Source: CAD feature listing. Evaluate the final solid. Frame: model axes, mm. Face numbers are marked on the shaded views. A direction names the side the tool comes from. Coordinates: 2 decimals unless noted, no trailing zeros. Order: outer loops, then holes, each group sorted by start corner. A loop starts at its lowest first (then second) coordinate and runs counter-clockwise, first axis right, second up.
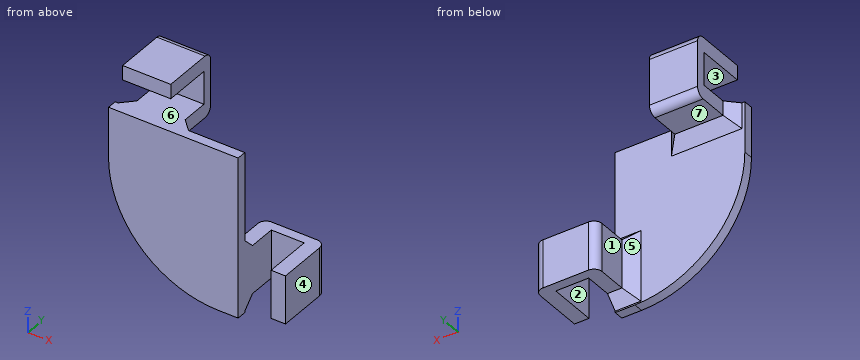
```python
from build123d import *

# Parameters (mm, degrees)
SKETCH1_W           = 30
SKETCH1_H           = 9
SKETCH1_W_2         = 9
SKETCH1_H_2         = 30
BOSS_EXTRUDE1_DEPTH = 6
BOSS_EXTRUDE2_START = 6
SKETCH1_3_W         = 30
SKETCH1_3_H         = 9
SKETCH1_3_W_2       = 9
SKETCH1_3_H_2       = 30
BOSS_EXTRUDE2_DEPTH = 24
BOSS_EXTRUDE3_START = 30
SKETCH1_4_W         = 30
SKETCH1_4_H         = 9
SKETCH1_4_H_2       = 20.5
SKETCH1_4_W_2       = 9
SKETCH1_4_H_3       = 30
SKETCH1_4_W_3       = 20.5
BOSS_EXTRUDE3_DEPTH = 6
BOSS_EXTRUDE4_START = 30
SKETCH1_5_W         = 30
SKETCH1_5_H         = 9
SKETCH1_5_W_2       = 9
SKETCH1_5_H_2       = 30
BOSS_EXTRUDE4_DEPTH = 30
CHAMFER1_SIZE       = 7
FILLET1_R           = 5


with BuildPart() as part:
    # Sketch1 → Boss-Extrude1 (new body)
    with BuildSketch(Plane(origin=(0, 0, 0), x_dir=(1, 0, 0), z_dir=(0, 1, 0))):
        with Locations((-57, 4.5)):
            Rectangle(SKETCH1_W, SKETCH1_H)
        with Locations((-4.5, 77)):
            Rectangle(SKETCH1_W_2, SKETCH1_H_2)
        with BuildLine():
            Line((0, 99.896112213), (-12.24628833, 99.896112213))
            ThreePointArc((-12.24628833, 99.896112213), (-60.703064532, 79.824658322), (-80.774518424, 31.36788212))
            Line((-80.774518424, 31.36788212), (-80.774518424, 0))
            Line((-80.774518424, 0), (-72, 0))
            Line((-72, 0), (-72, 9))
            Line((-72, 9), (-42, 9))
            Line((-42, 9), (-42, 0))
            Line((-42, 0), (0, 0))
            Line((0, 0), (0, 62))
            Line((0, 62), (-9, 62))
            Line((-9, 62), (-9, 92))
            Line((-9, 92), (0, 92))
            Line((0, 92), (0, 99.896112213))
        make_face()
    extrude(amount=BOSS_EXTRUDE1_DEPTH)

    # Sketch1<3> → Boss-Extrude2 (add)
    with BuildSketch(Plane(origin=(0, 0, 0), x_dir=(1, 0, 0), z_dir=(0, 1, 0)).offset(BOSS_EXTRUDE2_START)):
        with Locations((-57, 4.5)):
            Rectangle(SKETCH1_3_W, SKETCH1_3_H)
        with Locations((-4.5, 77)):
            Rectangle(SKETCH1_3_W_2, SKETCH1_3_H_2)
    extrude(amount=BOSS_EXTRUDE2_DEPTH)

    # Sketch1<4> → Boss-Extrude3 (add)
    with BuildSketch(Plane(origin=(0, 0, 0), x_dir=(1, 0, 0), z_dir=(0, 1, 0)).offset(BOSS_EXTRUDE3_START)):
        with Locations((-57, 4.5)):
            Rectangle(SKETCH1_4_W, SKETCH1_4_H)
        with Locations((-57, -10.25)):
            Rectangle(SKETCH1_4_W, SKETCH1_4_H_2)
        with Locations((-57, -25)):
            Rectangle(SKETCH1_4_W, SKETCH1_4_H)
        with Locations((-4.5, 77)):
            Rectangle(SKETCH1_4_W_2, SKETCH1_4_H_3)
        with Locations((10.25, 77)):
            Rectangle(SKETCH1_4_W_3, SKETCH1_4_H_3)
        with Locations((25, 77)):
            Rectangle(SKETCH1_4_W_2, SKETCH1_4_H_3)
    extrude(amount=BOSS_EXTRUDE3_DEPTH)

    # Sketch1<5> → Boss-Extrude4 (add)
    with BuildSketch(Plane(origin=(0, 0, 0), x_dir=(1, 0, 0), z_dir=(0, 1, 0)).offset(BOSS_EXTRUDE4_START)):
        with Locations((-57, -25)):
            Rectangle(SKETCH1_5_W, SKETCH1_5_H)
        with Locations((25, 77)):
            Rectangle(SKETCH1_5_W_2, SKETCH1_5_H_2)
    extrude(amount=-BOSS_EXTRUDE4_DEPTH)

    # Chamfer1
    chamfer1_edges = [part.edges().sort_by_distance(p)[0] for p in [
        (-42, 6, -4.5),
        (-72, 6, -4.5),
        (-57, 6, -9),
        (-4.5, 6, -92),
        (-4.5, 6, -62),
        (-9, 6, -77),
    ]]
    chamfer(chamfer1_edges, length=CHAMFER1_SIZE)

    # Fillet1
    fillet1_edges = [part.edges().sort_by_distance(p)[0] for p in [
        (-57, 36, -9),
        (-57, 36, 29.5),
        (29.5, 36, -77),
        (-9, 36, -77),
    ]]
    fillet(fillet1_edges, radius=FILLET1_R)


solid = part.part
```
1. Section query B-B on y = 19.5. Return loops of the section in (x, z), plus the area to 3 significant figures.
Findings:
outline: (-72, -9) - (-42, -9) - (-42, 0) - (-72, 0) - close; (-72, 20.5) - (-42, 20.5) - (-42, 29.5) - (-72, 29.5) - close; (-9, -92) - (0, -92) - (0, -62) - (-9, -62) - close; (20.5, -92) - (29.5, -92) - (29.5, -62) - (20.5, -62) - close
area: 1,080 mm2
2. Ray query, line 1 (X direction, y = 28.5, z = -80); line 2 (X direction, y = 34, z = 1.5). Return the intervals inside material, ascending.
Findings:
line 1: x = -9 to 0, 20.5 to 29.5
line 2: x = -72 to -42
3. Section query C-C on z = -10.5. Return loops of the section in (x, y).
Findings:
outline: (-80.77, 0) - (0, 0) - (0, 6) - (-35, 6) - (-40.5, 11.5) - (-73.5, 11.5) - (-79, 6) - (-80.77, 6) - close
4. Draft query along Z for the marked faces 5, 6 and 7. Return one class per face: released by +Z, released by -Z, zero draft, split by the parting line, or undercut.
Findings:
face 5: zero draft
face 6: undercut
face 7: released by -Z
5. Pin query (flat end, axial travel): P1, Ø14.5, axis at y = 23.5, z = -70, coming from the -X side; P2, Ø1.5, axis at y = 9.5, z = -63, coming from the -X side; P3, Ø10, axis at x = -22.5, z = -8, coming from the -Y side; P4, Ø18, axis at y = 17, z = 16, coming from the -X side. Return the tip coordinate at first contact, or that it passes through.
Findings:
P1: stops at x = -9
P2: stops at x = -13.25
P3: stops at y = 0
P4: stops at x = -72
6. Section query A-A on y = 4.5. Return loops of the section in (x, z).
Findings:
outline: (-80.77, -31.37) arc R68.53 ccw to (-12.25, -99.9) - (0, -99.9) - (0, 0) - (-80.77, 0) - close; (-72, 20.5) - (-42, 20.5) - (-42, 29.5) - (-72, 29.5) - close; (20.5, -92) - (29.5, -92) - (29.5, -62) - (20.5, -62) - close
7. Access query for the marked faces 1, 2, 3 and 4. Directions: +Z, -Z, +X, -X, +Y, -Y. A direction counts if a zero-diameter tool reaches every point of the face in a straight line with its end or side. Return the directions, or none.
Findings:
face 1: +Z, -Z, -X, +Y
face 2: +Z, -Z, -Y
face 3: +X, -X, -Y
face 4: +Z, -Z, +X, +Y, -Y
8. Section query D-D on x = -66. Return loops of the section in (y, z).
Findings:
outline: (0, -73.87) - (6, -73.87) - (6, -16) - (13, -9) - (31, -9) arc R5 ccw to (36, -4) - (36, 24.5) arc R5 ccw to (31, 29.5) - (0, 29.5) - (0, 20.5) - (30, 20.5) - (30, 0) - (0, 0) - close
